Geometry check sheet. Reference: the model listing, model coordinates, mm. Face numbers are marked on the shaded views. Coordinates: 2 decimals unless noted, no trailing zeros. Write each loop counter-clockwise with the first axis right and the second up, starting at its lowest first coordinate (ties: lowest second). Pieces come first, ordered by that corner, then holes. Notation, with made-up numbers: (3, 47.25) -> (56, 47.25) arc R28 ccw to (56, 72.25) -> close; hole circle Ø9 at (74.25, 51). An arc over 180 degrees is marked (long way). Use a Markdown table: item, result.
```python
from build123d import *

# Parameters (mm, degrees)
SKETCH2_R                   = 2.5
BOSS_EXTRUDE1_DEPTH         = 3
BOSS_EXTRUDE2_START         = 2.75
SKETCH3_W                   = 15
SKETCH3_H                   = 10
BOSS_EXTRUDE2_DEPTH         = 2.5
FILLET2_RADIUS              = 5
FILLET2_LENGTH              = 2.5
FILLET2_OF_MIRROR1_2_RADIUS = 5
FILLET2_OF_MIRROR1_2_LENGTH = 2.5
CHAMFER1_SIZE               = 2
CHAMFER2_SIZE               = 2
SKETCH5_R                   = 2.5
CUT_EXTRUDE2_DEPTH          = 68.694626818
CHAMFER3_SIZE               = 3
FILLET3_R                   = 2.5
CHAMFER4_SIZE               = 1
FILLET4_R                   = 30.5


with BuildPart() as part:
    # Sketch2 → Boss-Extrude1 (new body)
    with BuildSketch(Plane(origin=(0, 0, 0), x_dir=(1, 0, 0), z_dir=(0, 1, 0))):
        with BuildLine():
            Line((60, 0), (-60, 0))
            Line((-60, 0), (-60, -12))
            Line((-60, -12), (-24.738633754, -12))
            ThreePointArc((-24.738633754, -12), (0, -6), (24.738633754, -12))
            Line((24.738633754, -12), (60, -12))
            Line((60, -12), (60, 0))
        make_face()
        with Locations(Location((-52.5, -6, 0), (0, 0, 270))):
            Circle(SKETCH2_R, mode=Mode.SUBTRACT)
        with Locations(Location((52.5, -6, 0), (0, 0, 270))):
            Circle(SKETCH2_R, mode=Mode.SUBTRACT)
    extrude(amount=BOSS_EXTRUDE1_DEPTH)

    # Sketch3 → Boss-Extrude2 (add)
    with BuildSketch(Plane(origin=(0, 0, 0), x_dir=(0, 0, -1), z_dir=(1, 0, 0)).offset(BOSS_EXTRUDE2_START)):
        with Locations((7.5, 5)):
            Rectangle(SKETCH3_W, SKETCH3_H)
    boss_extrude2 = extrude(amount=BOSS_EXTRUDE2_DEPTH)

    # Fillet2: full round fillet: the end face becomes a half cylinder, R = half its width
    fillet2_face = Plane((4, 5, -15), x_dir=(-1, 0, 0), z_dir=(0, 0, -1))  # on the end face: x along it, z out of the body
    fillet2_slab = fillet2_face.offset(-FILLET2_RADIUS / 2) * Box(FILLET2_LENGTH, 2 * FILLET2_RADIUS, FILLET2_RADIUS, mode=Mode.PRIVATE)  # the body's end, R deep
    fillet2_round = Plane((4, 5, -10), x_dir=(0, 0, -1), z_dir=(-1, 0, 0)) * Cylinder(FILLET2_RADIUS, FILLET2_LENGTH, mode=Mode.PRIVATE)  # its axis R under the face
    add(fillet2_slab - fillet2_round, mode=Mode.SUBTRACT)

    # Mirror1: Boss-Extrude2 across plane
    add(boss_extrude2.mirror(Plane(origin=(0, 0, 0), x_dir=(0, 0, 1), z_dir=(1, 0, 0))))

    # Fillet2 of Mirror1 2: full round fillet: the end face becomes a half cylinder, R = half its width
    fillet2_of_mirror1_2_face = Plane((-4, 5, -15), x_dir=(1, 0, 0), z_dir=(0, 0, -1))  # on the end face: x along it, z out of the body
    fillet2_of_mirror1_2_slab = fillet2_of_mirror1_2_face.offset(-FILLET2_OF_MIRROR1_2_RADIUS / 2) * Box(FILLET2_OF_MIRROR1_2_LENGTH, 2 * FILLET2_OF_MIRROR1_2_RADIUS, FILLET2_OF_MIRROR1_2_RADIUS, mode=Mode.PRIVATE)  # the body's end, R deep
    fillet2_of_mirror1_2_round = Plane((-4, 5, -10), x_dir=(0, 0, -1), z_dir=(1, 0, 0)) * Cylinder(FILLET2_OF_MIRROR1_2_RADIUS, FILLET2_OF_MIRROR1_2_LENGTH, mode=Mode.PRIVATE)  # its axis R under the face
    add(fillet2_of_mirror1_2_slab - fillet2_of_mirror1_2_round, mode=Mode.SUBTRACT)

    # Chamfer1
    chamfer1_edges = [part.edges().sort_by_distance(p)[0] for p in [
        (4, 3, 0),
        (-4, 3, 0),
    ]]
    chamfer(chamfer1_edges, length=CHAMFER1_SIZE)

    # Chamfer2
    chamfer2_edges = [part.edges().sort_by_distance(p)[0] for p in [
        (-5.25, 1.5, 0),
        (5.25, 1.5, 0),
        (4, 10, 0),
        (-4, 10, 0),
    ]]
    chamfer(chamfer2_edges, length=CHAMFER2_SIZE)

    # Sketch5 → Cut-Extrude2 (cut, through all)
    with BuildSketch(Plane(origin=(5.25, 0, 0), x_dir=(0, 0, -1), z_dir=(1, 0, 0))):
        with Locations((10, 5)):
            Circle(SKETCH5_R)
    extrude(amount=-CUT_EXTRUDE2_DEPTH, mode=Mode.SUBTRACT)

    # Chamfer3
    chamfer3_edges = [part.edges().sort_by_distance(p)[0] for p in [
        (-60, 1.5, 12),
        (-60, 1.5, 0),
        (60, 1.5, 0),
        (60, 1.5, 12),
    ]]
    chamfer(chamfer3_edges, length=CHAMFER3_SIZE)

    # Fillet3
    fillet3_edges = [part.edges().sort_by_distance(p)[0] for p in [
        (-57, 1.5, 0),
        (-7.25, 1.5, 0),
        (-5.25, 1.5, -2),
        (-2.75, 1.5, 0),
        (2.75, 1.5, 0),
        (5.25, 1.5, -2),
        (7.25, 1.5, 0),
        (57, 1.5, 0),
        (60, 1.5, 3),
        (60, 1.5, 9),
        (57, 1.5, 12),
        (-60, 1.5, 3),
        (4, 8, 0),
        (4, 10, -2),
        (-4, 10, -2),
        (-4, 8, 0),
        (-60, 1.5, 9),
        (-57, 1.5, 12),
    ]]
    fillet(fillet3_edges, radius=FILLET3_R)

    # Chamfer4
    chamfer4_edges = [part.edges().sort_by_distance(p)[0] for p in [
        (-52.5, 3, 3.5),
        (52.5, 3, 3.5),
    ]]
    chamfer(chamfer4_edges, length=CHAMFER4_SIZE)

    # Fillet4
    fillet4_edges = [part.edges().sort_by_distance(p)[0] for p in [
        (-24.738633754, 1.5, 12),
        (24.738633754, 1.5, 12),
    ]]
    fillet(fillet4_edges, radius=FILLET4_R)


solid = part.part
```
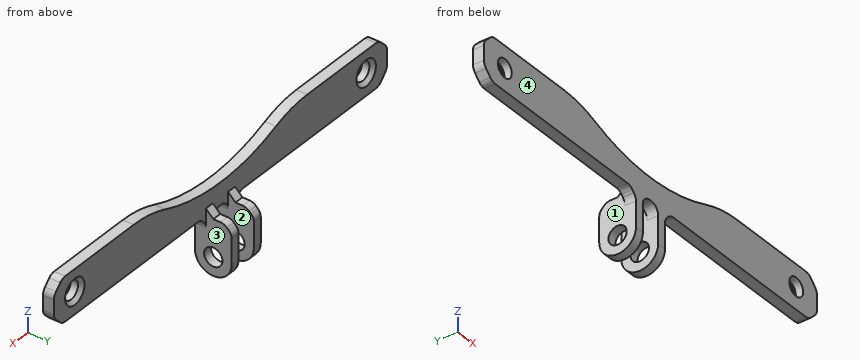
Item 1: Mould release check, pull along X, two halves, no side actions. Record for the marked faces 1, 2, 3 and 4: +X half, -X half, draft (parallel to the pull), parting line (faces both ways), or undercut.
Answer block:
| item | result |
|---|---|
| face 1 | -X half |
| face 2 | undercut |
| face 3 | +X half |
| face 4 | draft |
Item 2: Thickness scan on L1, parallel to X at y = 2.75, z = -12; L2, parallel to Y at x = -31.5, z = 6; L3, parallel to Z at x = 4.5, y = 6. Record the ranges inside material, lowest first. Write a range as [from, to].
Answer block:
| item | result |
|---|---|
| L1 | x = [-5.25, -2.75], [2.75, 5.25] |
| L2 | y = [0, 3] |
| L3 | z = [-14.9, -12.29], [-7.71, 0] |
Item 3: Section check A-A on x = -52.5. Record the boundary of the cut face in (y, z), then the cut area to 3 significant figures.
Answer block:
| item | result |
|---|---|
| outline | (0, 0) -> (3, 0) -> (3, 2.5) -> (2, 3.5) -> (0, 3.5) -> close; (0, 8.5) -> (2, 8.5) -> (3, 9.5) -> (3, 12) -> (0, 12) -> close |
| area | 20.0 mm^2 |
Item 4: Section check B-B on x = -16. Record the boundary of the cut face in (y, z), then the cut area to 3 significant figures.
Answer block:
| item | result |
|---|---|
| outline | (0, 0) -> (3, 0) -> (3, 8.42) -> (0, 8.42) -> close |
| area | 25.3 mm^2 |
Item 5: Section check C-C on x = 28. Record the boundary of the cut face in (y, z), then the cut area to 3 significant figures.
Answer block:
| item | result |
|---|---|
| outline | (0, 0) -> (3, 0) -> (3, 11.82) -> (0, 11.82) -> close |
| area | 35.5 mm^2 |
Item 6: Depth check by flat-ended pin: P1, Ø1.5, axis at x = -33.5, y = 1.5, coming from the -Z side; P2, Ø4.5, axis at x = 52.5, z = 6, coming from the +Y side; P3, Ø1.6, axis at x = -4, y = 6, coming from the +Z side; P4, Ø6, axis at y = 3, z = -10, coming from the +X side. Enter the tip coordinate at first touch or a pass-through.
Answer block:
| item | result |
|---|---|
| P1 | stops at z = 0 |
| P2 | passes through |
| P3 | stops at z = 0 |
| P4 | stops at x = 5.25 |
